Could you check a few things on this model? Use its own coordinates, in mm. A direction names the side the tool comes from. Give positions to 0.01 mm unless a question says otherwise; leave off trailing zeros. Order: outer loops, then holes, each group sorted by start corner. A loop starts at its lowest first (then second) coordinate and runs counter-clockwise, first axis right, second up.
(1) On a 3-axis mill with a long thin cutter (end or side, diameter ignored), from which of +Z, -Z, +X, -X, +Y, -Y can I reach the whole of each face in a straight line? I mean faces 4 (the cylindrical face through (4.751, 0.74, -16.285)), 5 (the cylindrical face through (14.925, 0.74, -42.315)), 6 (the cylindrical face through (9.04, 2.77, -46.69)). Say none if no direction works.
(2) Imagine slicing it at D-D, the plane z = -7.9. Write out the boundary of the cut face in (x, y) (3 decimals), then the cut area to 3 significant figures.
(3) If I drill on probe 1 along X at (y, z) = (3, -22.9) (3 decimals); probe 2 along X at (y, z) = (0.3, -40) (3 decimals); probe 3 along X at (y, z) = (2.75, -19.9) (3 decimals), over which ranges is the centre line in solid material (lowest first)?
(4) Imagine slicing it at A-A, the plane z = -13.9. Write out the boundary of the cut face in (x, y) (3 decimals), then the cut area to 3 significant figures.
(5) If we mould it in two halves opening along X, with no side actions, what happens to faces 1 (the flat face through (10, 3, 0)), 2 (the cylindrical face through (14.363, 3.965, -4.721)), 3 (the flat face through (0, 3, -16))? For each: released by +X, released by -X, zero draft, split by the parting line, or undercut.
(6) Imagine slicing it at B-B, the plane y = 3. State how many separate pieces and enclosed holes the cut face has, then the cut area to 3 significant figures.
(7) Will these pins go through, and if not, where does the flat tip stop? pin 1 (1.6 mm diameter, centred on x = 7, z = -22.9, fed in from -Y); pin 2 (2.5 mm diameter, centred on x = 3, z = -45, fed in from +Y); pin 3 (1.5 mm diameter, centred on x = 3.5, z = -15, fed in from -Y); pin 4 (3 mm diameter, centred on x = 23.5, y = 2, fed in from +Z).
from build123d import *

# Parameters (mm, degrees)
BOSS_EXTRUDE1_DEPTH = 4
SKETCH2_W           = 20
SKETCH2_H           = 28
BOSS_EXTRUDE2_DEPTH = 2.5
CUT_EXTRUDE1_REACH  = 61.611
SKETCH3_R           = 1.375
SKETCH3_R_2         = 1.275
SKETCH4_R           = 2.5
CUT_EXTRUDE2_DEPTH  = 1.5
SKETCH5_R           = 2.5
CUT_EXTRUDE3_DEPTH  = 2.5


with BuildPart() as part:
    # Sketch1 → Boss-Extrude1 (new body)
    with BuildSketch(Plane(origin=(0, 0, 0), x_dir=(1, 0, 0), z_dir=(0, 1, 0))):
        Polygon((0, 0), (20, 0), (20, 33), (26.5, 33), (26.5, 53), (-6.5, 53), (-6.5, 33), (0, 33), align=None)
    extrude(amount=BOSS_EXTRUDE1_DEPTH)

    # Sketch2 → Boss-Extrude2 (add)
    with BuildSketch(Plane(origin=(0, 4, 0), x_dir=(1, 0, 0), z_dir=(0, 1, 0))):
        with Locations((10, 14)):
            Rectangle(SKETCH2_W, SKETCH2_H)
    extrude(amount=BOSS_EXTRUDE2_DEPTH)

    # Sketch3 → Cut-Extrude1 (cut, up to next)
    with BuildSketch(Plane.XZ, mode=Mode.PRIVATE) as cut_extrude1_sk1:
        with Locations(Location((10, -7.9, 0), (0, 0, 270))):
            Circle(SKETCH3_R)
    cut_extrude1_tool1 = extrude(cut_extrude1_sk1.sketch, amount=-CUT_EXTRUDE1_REACH, mode=Mode.PRIVATE) & part.part
    # Sketch3 → Cut-Extrude1 (cut, up to next)
    with BuildSketch(Plane.XZ, mode=Mode.PRIVATE) as cut_extrude1_sk2:
        with Locations(Location((7, -4.9, 0), (0, 0, 270))):
            Circle(SKETCH3_R)
    cut_extrude1_tool2 = extrude(cut_extrude1_sk2.sketch, amount=-CUT_EXTRUDE1_REACH, mode=Mode.PRIVATE) & part.part
    # Sketch3 → Cut-Extrude1 (cut, up to next)
    with BuildSketch(Plane.XZ, mode=Mode.PRIVATE) as cut_extrude1_sk3:
        with Locations(Location((4, -13.9, 0), (0, 0, 270))):
            Circle(SKETCH3_R)
    cut_extrude1_tool3 = extrude(cut_extrude1_sk3.sketch, amount=-CUT_EXTRUDE1_REACH, mode=Mode.PRIVATE) & part.part
    # Sketch3 → Cut-Extrude1 (cut, up to next)
    with BuildSketch(Plane.XZ, mode=Mode.PRIVATE) as cut_extrude1_sk4:
        with Locations(Location((10, -19.9, 0), (0, 0, 270))):
            Circle(SKETCH3_R)
    cut_extrude1_tool4 = extrude(cut_extrude1_sk4.sketch, amount=-CUT_EXTRUDE1_REACH, mode=Mode.PRIVATE) & part.part
    # Sketch3 → Cut-Extrude1 (cut, up to next)
    with BuildSketch(Plane.XZ, mode=Mode.PRIVATE) as cut_extrude1_sk5:
        with Locations(Location((7, -22.9, 0), (0, 0, 270))):
            Circle(SKETCH3_R)
    cut_extrude1_tool5 = extrude(cut_extrude1_sk5.sketch, amount=-CUT_EXTRUDE1_REACH, mode=Mode.PRIVATE) & part.part
    # Sketch3 → Cut-Extrude1 (cut, up to next)
    with BuildSketch(Plane.XZ, mode=Mode.PRIVATE) as cut_extrude1_sk6:
        with Locations(Location((13, -4.9, 0), (0, 0, 270))):
            Circle(SKETCH3_R)
    cut_extrude1_tool6 = extrude(cut_extrude1_sk6.sketch, amount=-CUT_EXTRUDE1_REACH, mode=Mode.PRIVATE) & part.part
    # Sketch3 → Cut-Extrude1 (cut, up to next)
    with BuildSketch(Plane.XZ, mode=Mode.PRIVATE) as cut_extrude1_sk7:
        with Locations(Location((13, -22.9, 0), (0, 0, 270))):
            Circle(SKETCH3_R)
    cut_extrude1_tool7 = extrude(cut_extrude1_sk7.sketch, amount=-CUT_EXTRUDE1_REACH, mode=Mode.PRIVATE) & part.part
    # Sketch3 → Cut-Extrude1 (cut, up to next)
    with BuildSketch(Plane.XZ, mode=Mode.PRIVATE) as cut_extrude1_sk8:
        with Locations(Location((16, -13.9, 0), (0, 0, 270))):
            Circle(SKETCH3_R)
    cut_extrude1_tool8 = extrude(cut_extrude1_sk8.sketch, amount=-CUT_EXTRUDE1_REACH, mode=Mode.PRIVATE) & part.part
    # Sketch3 → Cut-Extrude1 (cut, up to next)
    with BuildSketch(Plane.XZ, mode=Mode.PRIVATE) as cut_extrude1_sk9:
        with Locations(Location((10, -49, 0), (0, 0, 270))):
            Circle(SKETCH3_R_2)
    cut_extrude1_tool9 = extrude(cut_extrude1_sk9.sketch, amount=-CUT_EXTRUDE1_REACH, mode=Mode.PRIVATE) & part.part
    # Sketch3 → Cut-Extrude1 (cut, up to next)
    with BuildSketch(Plane.XZ, mode=Mode.PRIVATE) as cut_extrude1_sk10:
        with Locations(Location((4, -43, 0), (0, 0, 270))):
            Circle(SKETCH3_R_2)
    cut_extrude1_tool10 = extrude(cut_extrude1_sk10.sketch, amount=-CUT_EXTRUDE1_REACH, mode=Mode.PRIVATE) & part.part
    # Sketch3 → Cut-Extrude1 (cut, up to next)
    with BuildSketch(Plane.XZ, mode=Mode.PRIVATE) as cut_extrude1_sk11:
        with Locations(Location((1, -46, 0), (0, 0, 270))):
            Circle(SKETCH3_R_2)
    cut_extrude1_tool11 = extrude(cut_extrude1_sk11.sketch, amount=-CUT_EXTRUDE1_REACH, mode=Mode.PRIVATE) & part.part
    # Sketch3 → Cut-Extrude1 (cut, up to next)
    with BuildSketch(Plane.XZ, mode=Mode.PRIVATE) as cut_extrude1_sk12:
        with Locations(Location((10, -37, 0), (0, 0, 90))):
            Circle(SKETCH3_R_2)
    cut_extrude1_tool12 = extrude(cut_extrude1_sk12.sketch, amount=-CUT_EXTRUDE1_REACH, mode=Mode.PRIVATE) & part.part
    # Sketch3 → Cut-Extrude1 (cut, up to next)
    with BuildSketch(Plane.XZ, mode=Mode.PRIVATE) as cut_extrude1_sk13:
        with Locations(Location((1, -40, 0), (0, 0, 90))):
            Circle(SKETCH3_R_2)
    cut_extrude1_tool13 = extrude(cut_extrude1_sk13.sketch, amount=-CUT_EXTRUDE1_REACH, mode=Mode.PRIVATE) & part.part
    # Sketch3 → Cut-Extrude1 (cut, up to next)
    with BuildSketch(Plane.XZ, mode=Mode.PRIVATE) as cut_extrude1_sk14:
        with Locations(Location((19, -46, 0), (0, 0, 90))):
            Circle(SKETCH3_R_2)
    cut_extrude1_tool14 = extrude(cut_extrude1_sk14.sketch, amount=-CUT_EXTRUDE1_REACH, mode=Mode.PRIVATE) & part.part
    # Sketch3 → Cut-Extrude1 (cut, up to next)
    with BuildSketch(Plane.XZ, mode=Mode.PRIVATE) as cut_extrude1_sk15:
        with Locations(Location((16, -43, 0), (0, 0, 90))):
            Circle(SKETCH3_R_2)
    cut_extrude1_tool15 = extrude(cut_extrude1_sk15.sketch, amount=-CUT_EXTRUDE1_REACH, mode=Mode.PRIVATE) & part.part
    # Sketch3 → Cut-Extrude1 (cut, up to next)
    with BuildSketch(Plane.XZ, mode=Mode.PRIVATE) as cut_extrude1_sk16:
        with Locations(Location((19, -40, 0), (0, 0, 270))):
            Circle(SKETCH3_R_2)
    cut_extrude1_tool16 = extrude(cut_extrude1_sk16.sketch, amount=-CUT_EXTRUDE1_REACH, mode=Mode.PRIVATE) & part.part
    add(cut_extrude1_tool1.solids().sort_by_distance((10, 0, -7.9))[0], mode=Mode.SUBTRACT)
    add(cut_extrude1_tool2.solids().sort_by_distance((7, 0, -4.9))[0], mode=Mode.SUBTRACT)
    add(cut_extrude1_tool3.solids().sort_by_distance((4, 0, -13.9))[0], mode=Mode.SUBTRACT)
    add(cut_extrude1_tool4.solids().sort_by_distance((10, 0, -19.9))[0], mode=Mode.SUBTRACT)
    add(cut_extrude1_tool5.solids().sort_by_distance((7, 0, -22.9))[0], mode=Mode.SUBTRACT)
    add(cut_extrude1_tool6.solids().sort_by_distance((13, 0, -4.9))[0], mode=Mode.SUBTRACT)
    add(cut_extrude1_tool7.solids().sort_by_distance((13, 0, -22.9))[0], mode=Mode.SUBTRACT)
    add(cut_extrude1_tool8.solids().sort_by_distance((16, 0, -13.9))[0], mode=Mode.SUBTRACT)
    add(cut_extrude1_tool9.solids().sort_by_distance((10, 0, -49))[0], mode=Mode.SUBTRACT)
    add(cut_extrude1_tool10.solids().sort_by_distance((4, 0, -43))[0], mode=Mode.SUBTRACT)
    add(cut_extrude1_tool11.solids().sort_by_distance((1, 0, -46))[0], mode=Mode.SUBTRACT)
    add(cut_extrude1_tool12.solids().sort_by_distance((10, 0, -37))[0], mode=Mode.SUBTRACT)
    add(cut_extrude1_tool13.solids().sort_by_distance((1, 0, -40))[0], mode=Mode.SUBTRACT)
    add(cut_extrude1_tool14.solids().sort_by_distance((19, 0, -46))[0], mode=Mode.SUBTRACT)
    add(cut_extrude1_tool15.solids().sort_by_distance((16, 0, -43))[0], mode=Mode.SUBTRACT)
    add(cut_extrude1_tool16.solids().sort_by_distance((19, 0, -40))[0], mode=Mode.SUBTRACT)

    # Sketch4 → Cut-Extrude2 (cut)
    with BuildSketch(Plane.XZ):
        with Locations(Location((4, -13.9, 0), (0, 0, 270))):
            Circle(SKETCH4_R)
        with Locations(Location((16, -13.9, 0), (0, 0, 270))):
            Circle(SKETCH4_R)
        with BuildLine():
            ThreePointArc((15.5, -22.9), (10, -17.4), (4.5, -22.9))
            ThreePointArc((4.5, -22.9), (7, -25.4), (9.5, -22.9))
            ThreePointArc((9.5, -22.9), (10, -22.4), (10.5, -22.9))
            ThreePointArc((10.5, -22.9), (13, -25.4), (15.5, -22.9))
        make_face()
        with BuildLine():
            ThreePointArc((15.5, -4.9), (10, -10.4), (4.5, -4.9))
            ThreePointArc((4.5, -4.9), (7, -2.4), (9.5, -4.9))
            ThreePointArc((9.5, -4.9), (10, -5.4), (10.5, -4.9))
            ThreePointArc((10.5, -4.9), (13, -2.4), (15.5, -4.9))
        make_face()
    extrude(amount=-CUT_EXTRUDE2_DEPTH, mode=Mode.SUBTRACT)

    # Sketch5 → Cut-Extrude3 (cut)
    with BuildSketch(Plane(origin=(0, 4, 0), x_dir=(1, 0, 0), z_dir=(0, 1, 0))):
        with Locations(Location((10, 49, 0), (0, 0, 270))):
            Circle(SKETCH5_R)
        with Locations(Location((10, 37, 0), (0, 0, 270))):
            Circle(SKETCH5_R)
        with BuildLine():
            ThreePointArc((19, 48.3), (13.7, 43), (19, 37.7))
            ThreePointArc((19, 37.7), (21.3, 40), (19, 42.3))
            ThreePointArc((19, 42.3), (18.3, 43), (19, 43.7))
            ThreePointArc((19, 43.7), (21.3, 46), (19, 48.3))
        make_face()
        with BuildLine():
            ThreePointArc((1, 48.3), (6.3, 43), (1, 37.7))
            ThreePointArc((1, 37.7), (-1.3, 40), (1, 42.3))
            ThreePointArc((1, 42.3), (1.7, 43), (1, 43.7))
            ThreePointArc((1, 43.7), (-1.3, 46), (1, 48.3))
        make_face()
    extrude(amount=-CUT_EXTRUDE3_DEPTH, mode=Mode.SUBTRACT)


solid = part.part
Answer block:
1. face 4: -Y
1. face 5: +Y, -Y
1. face 6: +Y
2. outline: (0, 0) - (5.39, 0) - (5.39, 1.5) - (8.625, 1.5) - (8.625, 6.5) - (0, 6.5) - close; (11.375, 1.5) - (14.61, 1.5) - (14.61, 0) - (20, 0) - (20, 6.5) - (11.375, 6.5) - close
2. area: 102 mm2
3. probe 1: x = 0 to 5.625, 8.375 to 11.625, 14.375 to 20
3. probe 2: x = -6.5 to -0.275, 2.275 to 17.725, 20.275 to 26.5
3. probe 3: x = 0 to 8.625, 11.375 to 20
4. outline: (0, 0) - (1.5, 0) - (1.5, 1.5) - (2.625, 1.5) - (2.625, 6.5) - (0, 6.5) - close; (5.375, 1.5) - (6.5, 1.5) - (6.5, 0) - (13.5, 0) - (13.5, 1.5) - (14.625, 1.5) - (14.625, 6.5) - (5.375, 6.5) - close; (17.375, 1.5) - (18.5, 1.5) - (18.5, 0) - (20, 0) - (20, 6.5) - (17.375, 6.5) - close
4. area: 87.5 mm2
5. face 1: zero draft
5. face 2: undercut
5. face 3: released by -X
6. separate pieces: 1
6. enclosed holes: 12
6. area: 1,110 mm2
7. pin 1: passes through
7. pin 2: stops at y = 1.5
7. pin 3: stops at y = 1.5
7. pin 4: stops at z = -33
